Check sheet for the modelled part. Datum: model origin and axes. Units: mm. Coordinates: 2 decimals unless noted, no trailing zeros. Loops run counter-clockwise (first coordinate to the right, second up) from the corner with the lowest first, then second, coordinate; pieces in that order, holes last. Notation, with made-up numbers: (44.5, -18.75) - (77.5, -18.75) arc R31 ccw to (77.5, 15.25) - close; hole circle Ø10 at (7.5, 38). An arc over 180 degrees is marked (long way). Use a Markdown table: item, result. Add a question column.
1) Sectioned sample at B-B, the plane x = 42. Enter the section's corners in (y, z), then the cut area to 3 significant figures.
2) Thickness scan on line 1 (Z direction, x = 42, y = 2.35); line 2 (Z direction, x = 28, y = 8.5); line 3 (X direction, y = 6.75, z = 6). Record the ranges inside material, lowest first.
3) Sectioned sample at A-A, the plane z = 6. Enter the section's corners in (x, y).
4) Sectioned sample at C-C, the plane y = 7.5. Enter the section's corners in (x, z).
5) Go/stop test with flat-tipped pins: P1, Ø4, axis at x = 28, z = 6, coming from the -Y side; P2, Ø2, axis at x = 18, z = 3.5, coming from the +Y side. Record where each tip stops, or that it passes through.
6) Draft check along Z on faces 1 (the cylindrical face through (29.84, 7.34, 7.69)), 2 (the flat face through (2, 14, 6)), 3 (the flat face through (41, 4, 0)). Enter one of: pulls with the +Z half, pulls with the -Z half, needs draft (parallel to the pull), parting line crosses it, or undercut.
7) Sectioned sample at D-D, the plane y = 3. Enter the section's corners in (x, z), then the cut area to 3 significant figures.
from build123d import *

# Parameters (mm, degrees)
SKETCH_W               = 84
SKETCH_H               = 14
PAD_DEPTH              = 12
SKETCH001_R            = 9.75
POCKET_DEPTH           = 12.001
LINEARPATTERN001_COUNT = 3
LINEARPATTERN001_PITCH = 28
HOLE_D                 = 5
HOLE_CSINK_D           = 6
HOLE_CSINK_ANGLE       = 90
LINEARPATTERN_COUNT    = 2
LINEARPATTERN_PITCH    = 28
SKETCH003_R            = 2.8
POCKET001_DEPTH        = 14.001


with BuildPart() as part:
    # Sketch → Pad (new body)
    with BuildSketch(Plane.XY):
        with Locations((42, 7)):
            Rectangle(SKETCH_W, SKETCH_H)
    extrude(amount=PAD_DEPTH)

    # Sketch001 (on DatumPlane) → Pocket (cut, through all)
    with BuildSketch(Plane.XY.offset(12)):
        with Locations((14, 14)):
            Circle(SKETCH001_R)
    pocket = extrude(amount=-POCKET_DEPTH, mode=Mode.SUBTRACT)

    # LinearPattern001: Pocket ×3
    with Locations(*[(i * LINEARPATTERN001_PITCH, 0, 0) for i in range(1, LINEARPATTERN001_COUNT)]):
        add(pocket, mode=Mode.SUBTRACT)

    # Hole (through all)
    with Locations(Plane.XZ):
        with Locations((28, 6)):
            hole = CounterSinkHole(HOLE_D / 2, HOLE_CSINK_D / 2, counter_sink_angle=HOLE_CSINK_ANGLE)

    # LinearPattern: Hole ×2
    with Locations(*[(i * LINEARPATTERN_PITCH, 0, 0) for i in range(1, LINEARPATTERN_COUNT)]):
        add(hole, mode=Mode.SUBTRACT)

    # Sketch003 → Pocket001 (cut, through all)
    with BuildSketch(Plane.XZ):
        with Locations((42, 6)):
            Circle(SKETCH003_R)
    extrude(amount=-POCKET001_DEPTH, mode=Mode.SUBTRACT)


solid = part.part
Solved:
| question | item | result |
|---|---|---|
| 1 | outline | (0, 0) - (4.25, 0) - (4.25, 3.2) - (0, 3.2) - close; (0, 8.8) - (4.25, 8.8) - (4.25, 12) - (0, 12) - close |
| 1 | area | 27.2 mm2 |
| 2 | line 1 | z = 0 to 3.2, 8.8 to 12 |
| 2 | line 2 | z = 0 to 3.5, 8.5 to 12 |
| 2 | line 3 | x = 0 to 7.48, 20.52 to 25.5, 30.5 to 35.48, 48.52 to 53.5, 58.5 to 63.48, 76.52 to 84 |
| 3 | outline | (0, 0) - (25, 0) - (25.5, 0.5) - (25.5, 14) - (23.75, 14) arc R9.75 cw to (4.25, 14) - (0, 14) - close; (30.5, 0.5) - (31, 0) - (39.2, 0) - (39.2, 4.66) arc R9.75 cw to (32.25, 14) - (30.5, 14) - close; (44.8, 0) - (53, 0) - (53.5, 0.5) - (53.5, 14) - (51.75, 14) arc R9.75 cw to (44.8, 4.66) - close; (58.5, 0.5) - (59, 0) - (84, 0) - (84, 14) - (79.75, 14) arc R9.75 cw to (60.25, 14) - (58.5, 14) - close |
| 4 | outline | (0, 0) - (6.73, 0) - (6.73, 12) - (0, 12) - close; (21.27, 0) - (34.73, 0) - (34.73, 12) - (21.27, 12) - close; (49.27, 0) - (62.73, 0) - (62.73, 12) - (49.27, 12) - close; (77.27, 0) - (84, 0) - (84, 12) - (77.27, 12) - close; hole circle Ø5 at (28, 6); hole circle Ø5 at (56, 6) |
| 5 | P1 | passes through |
| 5 | P2 | stops at y = 5.63 |
| 6 | face 1 | undercut |
| 6 | face 2 | needs draft |
| 6 | face 3 | pulls with the -Z half |
| 7 | outline | (0, 0) - (84, 0) - (84, 12) - (0, 12) - close; hole circle Ø5 at (28, 6); hole circle Ø5.6 at (42, 6); hole circle Ø5 at (56, 6) |
| 7 | area | 944 mm2 |
